Check sheet for the modelled part. Datum: model origin and axes. Units: mm. Face numbers are marked on the shaded views. A direction names the side the tool comes from. Round coordinates to 2 decimals unless told otherwise and drop trailing zeros. Order: outer loops, then holes, each group sorted by start corner. A loop starts at its lowest first (then second) coordinate and runs counter-clockwise, first axis right, second up.
(1) Sectioned sample at A-A, the plane x = 0. Enter the section's corners in (y, z).
(2) Sectioned sample at D-D, the plane x = -48. Enter the section's corners in (y, z).
(3) Sectioned sample at C-C, the plane z = 16.5. Enter the section's corners in (x, y), and give its area (3 significant figures).
(4) Depth check by flat-ended pin: pin 1 (3.5 mm diameter, centred on y = 37, z = -13.5, fed in from -X); pin 2 (1.5 mm diameter, centred on x = -49.5, y = 55.5, fed in from +Z); pin 3 (16.5 mm diameter, centred on y = 63.5, z = 97, fed in from +X); pin 4 (6 mm diameter, centred on x = 69.5, y = 49, fed in from -Z). Enter the tip coordinate at first touch or a pass-through.
(5) Sectioned sample at B-B, the plane y = 13. Enter the section's corners in (x, z).
(6) Thickness scan on probe 1 along Z at (x, y) = (108, 36); probe 2 along X at (y, z) = (36.95, -36); probe 3 along Z at (x, y) = (0, 103). Record the ranges inside material, lowest first.
(7) Tool access check on the marked faces 1, 2, 3 and 4. Record the directions out of +Z, -Z, +X, -X, +Y, -Y that give a thin tool (end or side, any length) a straight path to the whole face; none if there is none.
(8) Mould release check, pull along Z, two halves, no side actions. Record for the marked faces 5, 6, 7 and 8: released by +Z, released by -Z, zero draft, split by the parting line, or undercut.
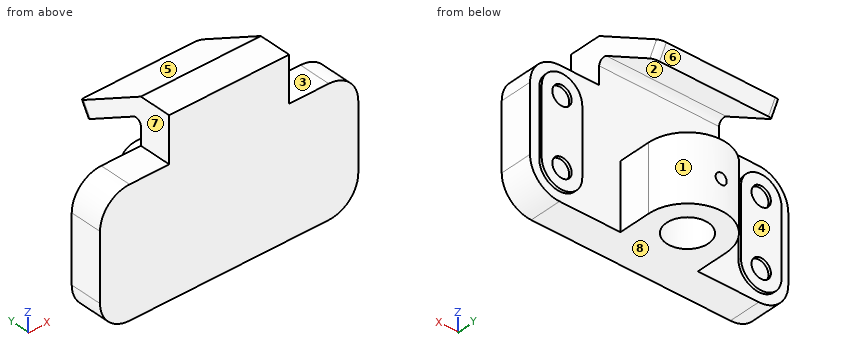
```python
from build123d import *

# Parameters (mm, degrees)
Y_KSEKLIK_EKSTR_ZYON1_DEPTH              = 35
IZIM3_R                                  = 10.5
Y_KSEKLIK_EKSTR_ZYON2_DEPTH              = 3
Y_KSEKLIK_EKSTR_ZYON3_DEPTH              = 71
IZIM5_R                                  = 11
KES_EKSTR_ZYON1_DEPTH                    = 21
IZIM6_R                                  = 6
KES_EKSTR_ZYON2_DEPTH                    = 23
M10_START                                = -68
M10_ALT_GEN_BA_L_C_VATA_IN_HAV_A1_OUTL_R = 22.5
M10_ALT_GEN_BA_L_C_VATA_IN_HAV_A1_DEPTH  = 50
IZIM9_W                                  = 130
IZIM9_H                                  = 35
Y_KSEKLIK_EKSTR_ZYON4_DEPTH              = 49
Y_KSEKLIK_EKSTR_ZYON5_DEPTH              = 130
RADYUS1_R                                = 6
RADYUS2_R                                = 6


# Read off the part's stored shape, not the designer's step: M10 Altıgen Başlı Cıvata İçin Havşa1
with BuildPart() as part:
    # Çizim1 → Yükseklik-Ekstrüzyon1 (new body)
    with BuildSketch(Plane(origin=(0, 0, 0), x_dir=(1, 0, 0), z_dir=(0, 1, 0))):
        with BuildLine():
            Line((-108, 68), (108, 68))
            ThreePointArc((108, 68), (130.627416998, 58.627416998), (140, 36))
            Line((140, 36), (140, -36))
            ThreePointArc((140, -36), (130.627416998, -58.627416998), (108, -68))
            Line((108, -68), (-108, -68))
            ThreePointArc((-108, -68), (-130.627416998, -58.627416998), (-140, -36))
            Line((-140, -36), (-140, 36))
            ThreePointArc((-140, 36), (-130.627416998, 58.627416998), (-108, 68))
        make_face()
    extrude(amount=Y_KSEKLIK_EKSTR_ZYON1_DEPTH)

    # Çizim3 → Yükseklik-Ekstrüzyon2 (add)
    # profile 1 of 2: a face of its own
    with BuildSketch(Plane(origin=(0, 35, 0), x_dir=(1, 0, 0), z_dir=(0, 1, 0))):
        with BuildLine():
            Line((-130, -36), (-130, 36))
            ThreePointArc((-130, 36), (-108, 58), (-86, 36))
            Line((-86, 36), (-86, -36))
            ThreePointArc((-86, -36), (-108, -58), (-130, -36))
        make_face()
        with Locations(Location((-108, 36, 0), (0, 0, 270))):
            Circle(IZIM3_R, mode=Mode.SUBTRACT)
        with Locations(Location((-108, -36, 0), (0, 0, 270))):
            Circle(IZIM3_R, mode=Mode.SUBTRACT)
    # profile 2 of 2: a face of its own
    with BuildSketch(Plane(origin=(0, 35, 0), x_dir=(1, 0, 0), z_dir=(0, 1, 0))):
        with BuildLine():
            Line((130, -36), (130, 36))
            ThreePointArc((130, 36), (108, 58), (86, 36))
            Line((86, 36), (86, -36))
            ThreePointArc((86, -36), (108, -58), (130, -36))
        make_face()
        with Locations(Location((108, -36, 0), (0, 0, 90))):
            Circle(IZIM3_R, mode=Mode.SUBTRACT)
        with Locations(Location((108, 36, 0), (0, 0, 90))):
            Circle(IZIM3_R, mode=Mode.SUBTRACT)
    extrude(amount=Y_KSEKLIK_EKSTR_ZYON2_DEPTH)

    # Çizim4 → Yükseklik-Ekstrüzyon3 (add)
    with BuildSketch(Plane(origin=(0, 0, -68), x_dir=(-1, 0, 0), z_dir=(0, 0, -1))):
        with BuildLine():
            Line((-42, 70), (-42, 35))
            Line((-42, 35), (42, 35))
            Line((42, 35), (42, 70))
            ThreePointArc((42, 70), (0, 112), (-42, 70))
        make_face()
    extrude(amount=-Y_KSEKLIK_EKSTR_ZYON3_DEPTH)

    # Çizim5 → Kes-Ekstrüzyon1 (cut)
    with BuildSketch(Plane.XY.offset(3)):
        with Locations((0, 70)):
            Circle(IZIM5_R)
    extrude(amount=-KES_EKSTR_ZYON1_DEPTH, mode=Mode.SUBTRACT)

    # Çizim6 → Kes-Ekstrüzyon2 (cut)
    with BuildSketch(Plane(origin=(0, 112, 0), x_dir=(1, 0, 0), z_dir=(0, 1, 0))):
        with Locations(Location((0, 36, 0), (0, 0, 270))):
            Circle(IZIM6_R)
    extrude(amount=-KES_EKSTR_ZYON2_DEPTH, mode=Mode.SUBTRACT)

    # M10 Altıgen Başlı Cıvata İçin Havşa1 outl → M10 Altıgen Başlı Cıvata İçin Havşa1 (cut)
    with BuildSketch(Plane.XY.offset(M10_START)):
        with Locations((0, 70)):
            Circle(M10_ALT_GEN_BA_L_C_VATA_IN_HAV_A1_OUTL_R)
    extrude(amount=M10_ALT_GEN_BA_L_C_VATA_IN_HAV_A1_DEPTH, mode=Mode.SUBTRACT)

    # Çizim9 → Yükseklik-Ekstrüzyon4 (add)
    with BuildSketch(Plane.XY.offset(68)):
        with Locations((0, 17.5)):
            Rectangle(IZIM9_W, IZIM9_H)
    extrude(amount=Y_KSEKLIK_EKSTR_ZYON4_DEPTH)

    # Çizim10 → Yükseklik-Ekstrüzyon5 (add)
    with BuildSketch(Plane(origin=(65, 0, 0), x_dir=(0, 0, -1), z_dir=(1, 0, 0))):
        Polygon((-117, 35), (-72.990557656, 111.226590152), (-58.413699339, 102.810637079), (-97.564188911, 35), align=None)
    extrude(amount=-Y_KSEKLIK_EKSTR_ZYON5_DEPTH)

    # Radyus1
    radyus1_edges = [part.edges().sort_by_distance(p)[0] for p in [
        (-65, 107.018613616, 65.702128498),
        (65, 107.018613616, 65.702128498),
    ]]
    fillet(radyus1_edges, radius=RADYUS1_R)

    # Radyus2
    radyus2_edges = [part.edges().sort_by_distance(p)[0] for p in [
        (0, 35, 97.564188911),
    ]]
    fillet(radyus2_edges, radius=RADYUS2_R)


solid = part.part
```
Derived:
1. outline: (0, -68) - (47.5, -68) - (47.5, -18) - (59, -18) - (59, 3) - (35, 3) - (35, 87.17) arc R6 cw to (44, 92.37) - (102.81, 58.41) - (111.23, 72.99) - (35, 117) - (0, 117) - close; (81, -18) - (92.5, -18) - (92.5, -30) - (112, -30) - (112, 3) - (81, 3) - close; (92.5, -68) - (112, -68) - (112, -42) - (92.5, -42) - close
2. outline: (0, -68) - (35, -68) - (35, 87.17) arc R6 cw to (44, 92.37) - (102.81, 58.41) - (111.23, 72.99) - (35, 117) - (0, 117) - close
3. outline: (-140, 0) - (140, 0) - (140, 35) - (130, 35) - (130, 38) - (86, 38) - (86, 35) - (-86, 35) - (-86, 38) - (-130, 38) - (-130, 35) - (-140, 35) - close
3. area: 10,100 mm2
4. pin 1: stops at x = -130
4. pin 2: stops at z = 105.6
4. pin 3: stops at x = 65
4. pin 4: passes through
5. outline: (-140, -36) arc R32 ccw to (-108, -68) - (108, -68) arc R32 ccw to (140, -36) - (140, 36) arc R32 ccw to (108, 68) - (65, 68) - (65, 117) - (-65, 117) - (-65, 68) - (-108, 68) arc R32 ccw to (-140, 36) - close
6. probe 1: z = -58 to -46.5, -25.5 to 25.5, 46.5 to 58
6. probe 2: x = -130 to -118.5, -97.5 to -86, -42 to 42, 86 to 97.5, 118.5 to 130
6. probe 3: z = -68 to -42, -30 to 3, 58.74 to 77.74
7. face 1: -Z, +Y
7. face 2: +X, -X
7. face 3: +Z, +X, +Y, -Y
7. face 4: +Z, -Z, -X, +Y
8. face 5: released by +Z
8. face 6: undercut
8. face 7: zero draft
8. face 8: released by -Z
